Build history of the part. All positions in model axes, mm. Face numbers are marked on the shaded views. A direction names the side the tool comes from. Give positions to 0.01 mm unless a question says otherwise; leave off trailing zeros. Order: outer loops, then holes, each group sorted by start corner. A loop starts at its lowest first (then second) coordinate and runs counter-clockwise, first axis right, second up. Notation, with made-up numbers: (-29, 47) -> (-18, 47) arc R12 ccw to (-18, 61) -> close; hole circle Ø3 at (35.5, 84.5). An arc over 180 degrees is marked (long way). One line per question, with ' | ' between items. Start each with the question number.
(1) Pin check, flat tips, straight feed: pin 1 Ø4 at (x, y) = (-21, -19.5) entering from +Z; pin 2 Ø2 at (x, z) = (49, 46) entering from +Y; pin 3 Ø3 at (x, y) = (50, 14) entering from +Z. Stop position of each tip, or through.
(2) Pull direction Y, two halves, no side cores. Call the marked faces 3, 4 and 5: +Y half, -Y half, draft (parallel to the pull), parting line (faces both ways), or undercut.
(3) Cut at D-D (y = -29.5). Give the cut face in (x, z), then the cut area to 3 significant figures.
(4) Cut at C-C (z = -1.5). Give the cut face in (x, y).
(5) Cut at B-B (y = 47). Give the cut face in (x, z), then the cut area to 3 significant figures.
(6) Which spindle directions (+Z, -Z, +X, -X, +Y, -Y) get a long thin tool onto all of the face, cutting with end or side? Do the marked faces 1 and 2. Say none if no direction does.
(7) Drill centre lines: L1, parallel to X at y = 27, z = -7; L2, parallel to Z at x = 3, y = 40; L3, parallel to X at y = -19.5, z = 36. Where is each one in solid material? Low to high. Write a range as from..to.
(8) Cut at A-A (y = 27). Give the cut face in (x, z), then the cut area to 3 significant figures.
from build123d import *

# Parameters (mm, degrees)
F1_DEPTH = 63.5
F2_DEPTH = 25.4
F3_DEPTH = 12.7


with BuildPart() as f1:
    # F0 (on Front) → F1 (new body, symmetric)
    with BuildSketch(Plane.XZ):
        Polygon((33.25627, 18.030804), (-38.082272, 18.030804), (-38.082272, -18.030804), (38.082272, -18.030804), (38.082272, 18.030804), align=None)
    extrude(amount=F1_DEPTH, both=True)

    # F0 (on Front) → F2 (join, symmetric)
    with BuildSketch(Plane.XZ):
        with BuildLine():
            Line((33.25627, 38.202789), (33.25627, 18.030804))
            Line((33.25627, 18.030804), (38.082272, 18.030804))
            Line((38.082272, 18.030804), (38.082272, 38.202789))
            ThreePointArc((38.082272, 38.202789), (40.858393, 45.442439), (47.763245, 48.969819))
            Line((47.763245, 48.969819), (51.281622, 48.969819))
            Line((51.281622, 48.969819), (51.281622, 53.79582))
            Line((51.281622, 53.79582), (47.53053, 53.79582))
            ThreePointArc((47.53053, 53.79582), (37.363711, 48.772759), (33.25627, 38.202789))
        make_face()
    extrude(amount=F2_DEPTH, both=True)

    # F0 (on Front) → F3 (join, symmetric)
    with BuildSketch(Plane.XZ):
        with BuildLine():
            add(Edge.make_bspline(
                [(-38.082272, 18.030804), (-5.656304, 18.834018), (25.872232, 73.464645), (51.281622, 53.79582)],
                knots=[0, 0, 0, 0, 96.255087, 96.255087, 96.255087, 96.255087], degree=3))
            Line((-38.082272, 18.030804), (33.25627, 18.030804))
            Line((33.25627, 18.030804), (33.25627, 38.202789))
            ThreePointArc((33.25627, 38.202789), (37.363711, 48.772759), (47.53053, 53.79582))
            Line((47.53053, 53.79582), (51.281622, 53.79582))
        make_face()
    extrude(amount=F3_DEPTH, both=True)

    # F0 (on Front) → F4 (revolve)
    with BuildSketch(Plane.XZ):
        Polygon((84.119728, 60.463159), (67.652359, 60.463159), (67.676517, 48.969819), (67.700675, 37.476478), (84.119728, 37.476478), align=None)
    revolve(axis=Axis((51.281622, 0, 48.969819), (0, 0, 1)))


solid = f1.part
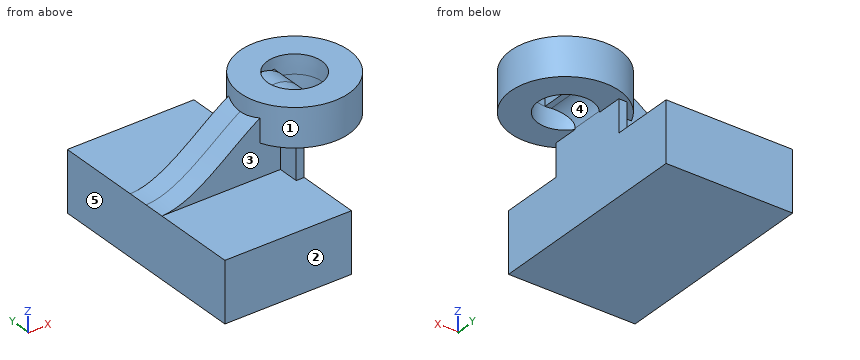
Result set:
1) pin 1: stops at z = 18.03 | pin 2: stops at y = 32.81 | pin 3: stops at z = 55.2
2) face 3: -Y half | face 4: undercut | face 5: draft
3) outline: (-38.08, -18.03) -> (38.08, -18.03) -> (38.08, 18.03) -> (-38.08, 18.03) -> close; (36.86, 37.48) -> (65.71, 37.48) -> (65.71, 60.46) -> (36.86, 60.46) -> close | area: 3,410 mm2
4) outline: (-38.08, -63.5) -> (38.08, -63.5) -> (38.08, 63.5) -> (-38.08, 63.5) -> close
5) outline: (-38.08, -18.03) -> (38.08, -18.03) -> (38.08, 18.03) -> (-38.08, 18.03) -> close | area: 2,750 mm2
6) face 1: +Z | face 2: +Z, -Z, +X, -X, -Y
7) L1: x = -38.08..38.08 | L2: z = -18.03..18.03 | L3: x = 33.26..38.08
8) outline: (-38.08, -18.03) -> (38.08, -18.03) -> (38.08, 18.03) -> (-38.08, 18.03) -> close; (32.59, 37.48) -> (69.97, 37.48) -> (69.97, 60.46) -> (32.59, 60.46) -> close | area: 3,610 mm2
